The figure shows three views and two pictorial views of one solid part (mm, origin at its lowest corner). Answer the questions. Coordinates: 2 decimals unless noted, no trailing zeros. Write each loop counter-clockwise with the first axis right and the second up, starting at its lowest first coordinate (ties: lowest second). Pieces come first, ordered by that corner, then holes.
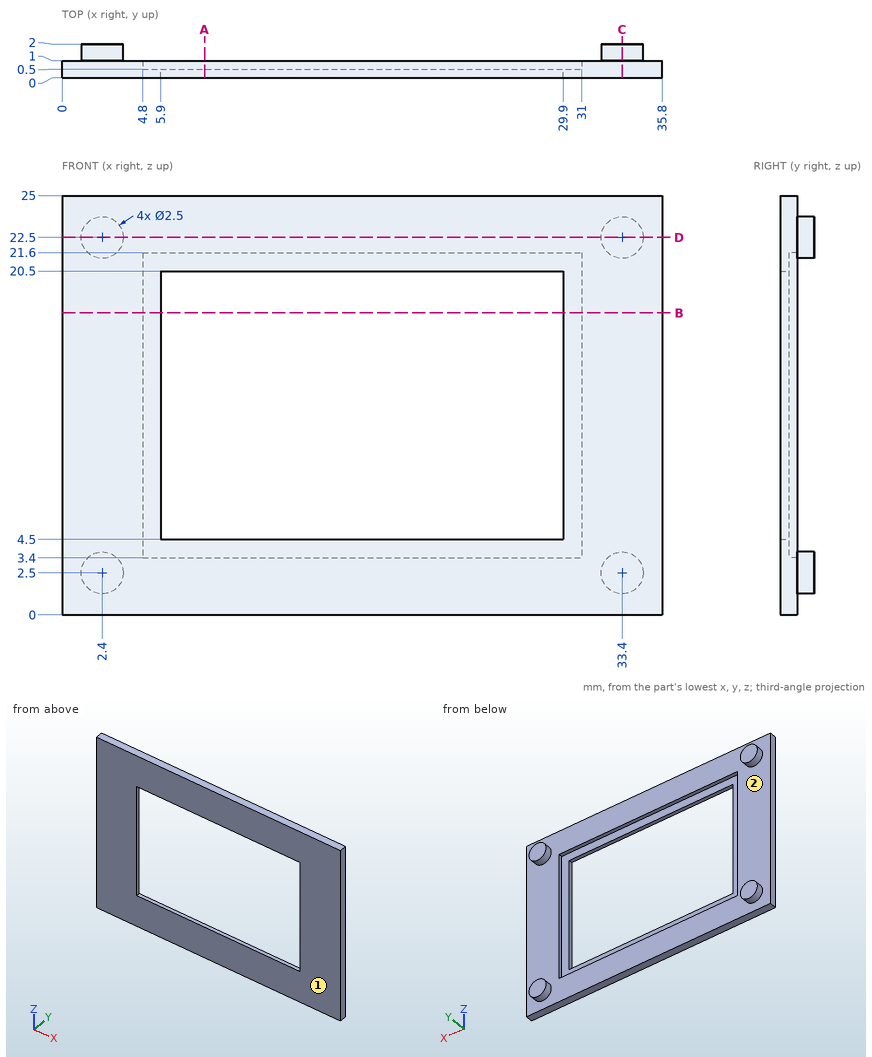
1. Section C-C on x = 33.4 is taken. Give the vertices of the cut face in (y, z), then the cut area to 3 significant figures.
Results found:
outline: (0, 0) - (1, 0) - (1, 1.25) - (2, 1.25) - (2, 3.75) - (1, 3.75) - (1, 21.25) - (2, 21.25) - (2, 23.75) - (1, 23.75) - (1, 25) - (0, 25) - close
area: 30.0 mm2
2. Section D-D on z = 22.5 is taken. Give the vertices of the cut face in (x, y), then the cut area to 3 significant figures.
Results found:
outline: (0, 0) - (35.8, 0) - (35.8, 1) - (34.65, 1) - (34.65, 2) - (32.15, 2) - (32.15, 1) - (3.65, 1) - (3.65, 2) - (1.15, 2) - (1.15, 1) - (0, 1) - close
area: 40.8 mm2
3. Section A-A on x = 8.5 is taken. Give the vertices of the cut face in (y, z), then the cut area to 3 significant figures.
Results found:
outline: (0, 0) - (1, 0) - (1, 3.4) - (0.5, 3.4) - (0.5, 4.5) - (0, 4.5) - close; (0, 20.5) - (0.5, 20.5) - (0.5, 21.6) - (1, 21.6) - (1, 25) - (0, 25) - close
area: 7.90 mm2
4. For a pull along X with two mould halves and no side action, classify the marked faces 1 and 2 as pulls with the +X half, pulls with the -X half, needs draft (parallel to the pull), parting line crosses it, or undercut.
Results found:
face 1: needs draft
face 2: undercut
5. Section B-B on z = 18 is taken. Give the vertices of the cut face in (x, y).
Results found:
outline: (0, 0) - (5.9, 0) - (5.9, 0.5) - (4.8, 0.5) - (4.8, 1) - (0, 1) - close; (29.9, 0) - (35.8, 0) - (35.8, 1) - (31, 1) - (31, 0.5) - (29.9, 0.5) - close
6. Find the intervals of material crossed by L1, parallel to X at y = 0.6, z = 5.5; L2, parallel to X at y = 0.15, z = 11.75; L3, parallel to Z at x = 21.5, y = 0.6, in increasing order.
Results found:
L1: x = 0 to 4.8, 31 to 35.8
L2: x = 0 to 5.9, 29.9 to 35.8
L3: z = 0 to 3.4, 21.6 to 25
7. A flat-ended cylindrical pin translates along its axis: P1, Ø8, axis at x = 29, z = 14.5, coming from the +Y side. Find the tip coordinate at first contact, or state that the pin passes through.
Results found:
P1: stops at y = 1
